```python
from build123d import *

# Parameters (mm, degrees)
F0_W     = 200
F0_H     = 100
F0_R     = 13.327869
F0_R_2   = 10
F1_DEPTH = 172


with BuildPart() as f1:
    # F0 (on Front) → F1 (new body)
    with BuildSketch(Plane.XZ):
        with Locations((100, -50)):
            Rectangle(F0_W, F0_H)
        with Locations((176.942766, -67.431971)):
            Circle(F0_R, mode=Mode.SUBTRACT)
        Polygon((80.127939, -50), (89.730337, -33.368159), (108.935133, -33.368159), (118.537531, -50), (108.935133, -66.631841), (89.730337, -66.631841), align=None, mode=Mode.SUBTRACT)
        with Locations((29.121823, -24.228896)):
            Circle(F0_R_2, mode=Mode.SUBTRACT)
    extrude(amount=F1_DEPTH)


solid = f1.part
```
Here's how the part is built. I have some questions about the finished solid (model axes, mm). A direction names the side the tool comes from. Coordinates: 2 decimals unless noted, no trailing zeros. Write each loop counter-clockwise with the first axis right and the second up, starting at its lowest first coordinate (ties: lowest second). Pieces come first, ordered by that corner, then holes. Notation, with made-up numbers: M 66.25,-30 L 106.25,-30 A29 ccw 106.25,-10 Z; hole C 39.25,14.25 d1. An arc over 180 degrees is marked long. Answer as CSV lines item,"result". Start each with the question number.
Q1. Suppose I cut it at A-A, the plane x = 94. List the corners of the cut face in (y, z) for me, then the cut area to 3 significant figures.
Q2. Suppose I cut it at B-B, the plane y = -36.5. List the corners of the cut face in (x, z) for me, then the cut area to 3 significant figures.
Q3. Will this pin go through, and if not, where does the flat tip stop? pin 1 Ø16 at (x, z) = (176.94, -67.43) entering from -Y.
Q4. For faces 1 (the flat face through (84.996, -84.796, -58.432)), 2 (the flat face through (0, -85, -51)), which set-ups out of +Z, -Z, +X, -X, +Y, -Y let a thin tool reach every point of the face, with its end or its side?
Q5. If we mould it in two halves opening along Z, with no side actions, what happens to faces 3 (the flat face through (76, 0, -49)), 4 (the flat face through (99, -85, 0)), 5 (the flat face through (113.804, -84.796, -58.199))? For each: pulls with the +Z half, pulls with the -Z half, needs draft (parallel to the pull), parting line crosses it, or undercut.
Q6. I need wall thicknesses on probe 1 along X at (y, z) = (-125, -26); probe 2 along X at (y, z) = (-52, -36); probe 3 along Z at (x, y) = (38, -161.5). Which ranges of each line are inside material? Lowest first, please. Write a range as [from, to].
Entries:
1,outline,"M -172,-100 L 0,-100 L 0,-66.63 L -172,-66.63 Z; M -172,-33.37 L 0,-33.37 L 0,0 L -172,0 Z"
1,area,"11,500 mm²"
2,outline,"M 0,-100 L 200,-100 L 200,0 L 0,0 Z; hole C 29.12,-24.23 d20; hole M 80.13,-50 L 89.73,-66.63 L 108.94,-66.63 L 118.54,-50 L 108.94,-33.37 L 89.73,-33.37 Z; hole C 176.94,-67.43 d26.66"
2,area,"18,200 mm²"
3,pin 1,"passes through"
4,face 1,"+Y, -Y"
4,face 2,"+Z, -Z, -X, +Y, -Y"
5,face 3,"needs draft"
5,face 4,"pulls with the +Z half"
5,face 5,"undercut"
6,probe 1,"x = [0, 19.28], [38.96, 200]"
6,probe 2,"x = [0, 88.21], [110.45, 200]"
6,probe 3,"z = [-100, -28.83], [-19.63, 0]"
